```python
from build123d import *

# Parameters (mm, degrees)
BOSS_EXTRUDE1_DEPTH = 1.5875
BOSS_EXTRUDE2_DEPTH = 1
FILLET1_R           = 2.54


with BuildPart() as part:
    # Sketch1 → Boss-Extrude1 (new body)
    with BuildSketch(Plane.XY):
        Polygon((40, 50), (-40, 50), (-40, 48), (-48, 48), (-48, 40), (-50, 40), (-50, -37.864895224), (-50, -40), (-48, -40), (-48, -48), (-40, -48), (-40, -50), (-37.864895224, -50), (40, -50), (40, -48), (48, -48), (48, -40), (50, -40), (50, 40), (48, 40), (48, 48), (40, 48), align=None)
    extrude(amount=BOSS_EXTRUDE1_DEPTH)

    # Sketch2 → Boss-Extrude2 (add)
    with BuildSketch(Plane.XY.offset(1.5875)):
        Polygon((-28.661165235, 45), (28.661165235, 45), (37.5, 36.161165235), (37.5, 25), (-37.5, 25), (-37.5, 36.161165235), align=None)
        Polygon((-28.661165235, 21.666666667), (28.661165235, 21.666666667), (37.5, 12.827831902), (37.5, 1.666666667), (-37.5, 1.666666667), (-37.5, 12.827831902), align=None)
        Polygon((-28.661165235, -1.666666667), (28.661165235, -1.666666667), (37.5, -10.505501431), (37.5, -21.666666667), (-37.5, -21.666666667), (-37.5, -10.505501431), align=None)
        Polygon((-37.5, -36.161165235), (-28.661165235, -45), (28.661165235, -45), (37.5, -36.161165235), (37.5, -25), (-37.5, -25), align=None)
    extrude(amount=BOSS_EXTRUDE2_DEPTH)

    # Fillet1
    # the kernel refuses this fillet: 2.54 mm, written as the material it adds along each edge
    with BuildSketch(Plane(origin=(-48, -40, 0), x_dir=(-1.0, -3.6735059438767946e-12, 0), z_dir=(0, 0, 1)), Plane(origin=(40, -48, 0), x_dir=(3.808509063671012e-12, -1.0, 0), z_dir=(0, 0, 1)), Plane(origin=(48, 40, 0), x_dir=(1.0, 3.659295089161617e-12, 0), z_dir=(0, 0, 1)), Plane(origin=(-40, 48, 0), x_dir=(-3.7978509226345916e-12, 1.0, 0), z_dir=(0, 0, 1))) as fillet1_piece_1:
        with BuildLine():
            CenterArc((2.54, 2.481934729), FILLET1_R, 180, 77.725329785)
            Line((0, 2.481934729), (-0.0508, 2.481934729))
            Line((-0.0508, 2.481934729), (-0.0508, 0))
            Line((-0.0508, 0), (0, -0.0508))
            ThreePointArc((0, -0.0508), (1, -0.0508), (1.9892, -0.049638695))
            Line((1.9892, -0.049638695), (2, 0))
        make_face()
    extrude(amount=1.5875)
    with BuildSketch(Plane(origin=(-40, -48, 0), x_dir=(-1, 0, 0), z_dir=(0, 0, 1)), Plane(origin=(48, -40, 0), x_dir=(0, -1, 0), z_dir=(0, 0, 1)), Plane(origin=(-48, 40, 0), x_dir=(0, 1, 0), z_dir=(0, 0, 1))) as fillet1_piece_2:
        with BuildLine():
            CenterArc((2.481934729, 2.54), FILLET1_R, 192.274670215, 77.725329785)
            Line((0, 2), (-0.049638695, 1.9892))
            ThreePointArc((-0.049638695, 1.9892), (-0.0508, 1), (-0.0508, 0))
            Line((-0.0508, 0), (0, -0.0508))
            Line((0, -0.0508), (2.481934729, -0.0508))
            Line((2.481934729, -0.0508), (2.481934729, 0))
        make_face()
    extrude(amount=1.5875)
    with BuildSketch(Plane(origin=(40, 48, 0), x_dir=(3.726796649058746e-12, 1.0, 0), z_dir=(0, 0, 1))) as fillet1_piece_3:
        with BuildLine():
            CenterArc((2.54, -2.481934729), FILLET1_R, 102.274670215, 77.725329785)
            Line((0, -2.481934729), (-0.0508, -2.481934729))
            Line((-0.0508, -2.481934729), (-0.0508, 0))
            Line((-0.0508, 0), (0, 0.0508))
            ThreePointArc((0, 0.0508), (1, 0.0508), (1.9892, 0.049638695))
            Line((1.9892, 0.049638695), (2, 0))
        make_face()
    extrude(amount=1.5875)


solid = part.part
```
Can you work these out from the model? Positions are in its coordinate system, mm. A direction names the side the tool comes from. Give positions to 0.01 mm unless a question says otherwise; leave off trailing zeros. Loops run counter-clockwise (first coordinate to the right, second up) from the corner with the lowest first, then second, coordinate; pieces in that order, holes last. Notation, with made-up numbers: M 36.25,-1.5 L 61.25,-1.5 A21 cw 61.25,24.5 Z; hole C 35.5,39.25 d2. An arc over 180 degrees is marked long. Answer in a Markdown table with one row per item.
1. Suppose I cut it at C-C on x = -9.5. Write out the boundary of the cut face in (y, z).
Taken from the geometry:
| item | result |
|---|---|
| outline | M -50,0 L 50,0 L 50,1.59 L 45,1.59 L 45,2.59 L 25,2.59 L 25,1.59 L 21.67,1.59 L 21.67,2.59 L 1.67,2.59 L 1.67,1.59 L -1.67,1.59 L -1.67,2.59 L -21.67,2.59 L -21.67,1.59 L -25,1.59 L -25,2.59 L -45,2.59 L -45,1.59 L -50,1.59 Z |
2. For pin 1 Ø0.5 at (x, z) = (-45.5, 1) entering from +Y; pin 2 Ø2 at (x, y) = (-40, -1.5) entering from +Z; pin 3 Ø0.8 at (y, z) = (44, 1) entering from -X, each with a flat end and sliding along its axis, tell me the tip position at first contact or that it passes through.
Taken from the geometry:
| item | result |
|---|---|
| pin 1 | stops at y = 48 |
| pin 2 | stops at z = 1.59 |
| pin 3 | stops at x = -48 |
3. Suppose I cut it at A-A on y = 8.5. Write out the boundary of the cut face in (x, z).
Taken from the geometry:
| item | result |
|---|---|
| outline | M -50,0 L 50,0 L 50,1.59 L 37.5,1.59 L 37.5,2.59 L -37.5,2.59 L -37.5,1.59 L -50,1.59 Z |
4. If I drill on line 1 along Y through (x, z) = (19, 2.4); line 2 along Y through (x, z) = (30.5, 2); line 3 along X through (y, z) = (-14.5, 1.85), over which ranges is the centre line in solid material (lowest first)?
Taken from the geometry:
| item | result |
|---|---|
| line 1 | y = -45 to -25, -21.67 to -1.67, 1.67 to 21.67, 25 to 45 |
| line 2 | y = -43.16 to -25, -21.67 to -3.51, 1.67 to 19.83, 25 to 43.16 |
| line 3 | x = -37.5 to 37.5 |
5. Suppose I cut it at D-D on y = -5.5. Write out the boundary of the cut face in (x, z), plus the area to 3 significant figures.
Taken from the geometry:
| item | result |
|---|---|
| outline | M -50,0 L 50,0 L 50,1.59 L 32.49,1.59 L 32.49,2.59 L -32.49,2.59 L -32.49,1.59 L -50,1.59 Z |
| area | 224 mm² |
6. Suppose I cut it at B-B on x = -30. Write out the boundary of the cut face in (y, z).
Taken from the geometry:
| item | result |
|---|---|
| outline | M -50,0 L 50,0 L 50,1.59 L 43.66,1.59 L 43.66,2.59 L 25,2.59 L 25,1.59 L 20.33,1.59 L 20.33,2.59 L 1.67,2.59 L 1.67,1.59 L -3.01,1.59 L -3.01,2.59 L -21.67,2.59 L -21.67,1.59 L -25,1.59 L -25,2.59 L -43.66,2.59 L -43.66,1.59 L -50,1.59 Z |
7. Which directions (+Z, -Z, +X, -X, +Y, -Y) give clear straight access to the entire face, cutting with the end or side of a thin tool? Please do faces 1 (the flat face through (33.02, 17.31, 2.08)), 2 (the flat face through (33.02, 40.64, 2.08)), 3 (the flat face through (33.02, -40.64, 2.08)).
Taken from the geometry:
| item | result |
|---|---|
| face 1 | +Z, +X |
| face 2 | +Z, +X, +Y |
| face 3 | +Z, +X, -Y |
8. Thinking about a two-plate mould opening in Y: for faces 4 (the flat face through (33.019, -6.024, 2.08)), 5 (the flat face through (1, 35, 2.588)), 6 (the flat face through (-33.14, 40.52, 2.08)), which applies, released by +Y, released by -Y, zero draft, split by the parting line, or undercut?
Taken from the geometry:
| item | result |
|---|---|
| face 4 | undercut |
| face 5 | zero draft |
| face 6 | released by +Y |
